```python
from build123d import *

# Parameters (mm, degrees)
F1_DEPTH  = 2
F3_DEPTH  = 3
F4_W      = 114.8
F4_H      = 24.2
F5_DEPTH  = 2
F7_DEPTH  = 2.2
F8_W      = 114.8
F8_H      = 2
F9_DEPTH  = 1
F10_W     = 114.8
F10_H     = 2
F11_DEPTH = 1
F12_DEPTH = 2


with BuildPart() as f1:
    # F0 (on Top) → F1 (new body)
    with BuildSketch(Plane.XY):
        Polygon((0, 40.2), (0, 0), (118.8, 0), (118.8, 40.2), (120.9, 40.2), (120.9, 155.2), (-2.1, 155.2), (-2.1, 40.2), align=None)
    extrude(amount=F1_DEPTH)

    # F2 (on face) → F3 (join)
    with BuildSketch(Plane.XY.offset(2)):
        Polygon((-2.1, 40.2), (0, 40.2), (0, 0), (118.8, 0), (118.8, 40.2), (120.9, 40.2), (120.9, 155.2), (-2.1, 155.2), align=None)
        Polygon((2, 42.2), (-0.1, 42.2), (-0.1, 153.2), (118.9, 153.2), (118.9, 42.2), (116.8, 42.2), (116.8, 2), (2, 2), align=None, mode=Mode.SUBTRACT)
    extrude(amount=F3_DEPTH)

    # F4 (on face) → F5 (join)
    with BuildSketch(Plane.XY.offset(2)):
        with Locations((59.4, 30.1)):
            Rectangle(F4_W, F4_H)
        Polygon((-0.1, 42.2), (2, 42.2), (59.4, 95.741176), (116.8, 42.2), (118.9, 42.2), (59.4, 97.7), align=None)
        Polygon((59.4, 97.7), (118.9, 42.2), (118.9, 44.158265), (61.499401, 97.7), (118.9, 151.241735), (118.9, 153.2), align=None)
        Polygon((-0.1, 153.2), (59.4, 97.7), (118.9, 153.2), (116.800599, 153.2), (59.4, 99.658265), (1.999401, 153.2), align=None)
        Polygon((-0.1, 44.158265), (-0.1, 42.2), (59.4, 97.7), (-0.1, 153.2), (-0.1, 151.241735), (57.300599, 97.7), align=None)
    extrude(amount=F5_DEPTH)

    # F6 (on face) → F7 (cut)
    with BuildSketch(Plane(origin=(0, 0, 0), x_dir=(1, 0, 0), z_dir=(0, 0, -1))):
        Polygon((0, -40.3), (118.8, -40.3), (118.8, -40.2), (118.8, -20.1), (0, -20.1), (0, -40.2), align=None)
    extrude(amount=-F7_DEPTH, mode=Mode.SUBTRACT)

    # F8 (on face) → F9 (cut)
    with BuildSketch(Plane.XY.offset(5)):
        with Locations((59.4, 1)):
            Rectangle(F8_W, F8_H)
    extrude(amount=-F9_DEPTH, mode=Mode.SUBTRACT)

    # F10 (on face) → F11 (cut)
    with BuildSketch(Plane.XY.offset(5)):
        with Locations((59.4, 154.2)):
            Rectangle(F10_W, F10_H)
    extrude(amount=-F11_DEPTH, mode=Mode.SUBTRACT)

    # F7_face (on face) → F12 (join)
    with BuildSketch(Plane(origin=(59.4, 97.748291, 0), x_dir=(1, 0, 0), z_dir=(0, 0, -1))):
        Polygon((-59.4, 57.548291), (-61.5, 57.548291), (-61.5, -57.451709), (61.5, -57.451709), (61.5, 57.548291), (59.4, 57.548291), (59.4, 57.448291), (-59.4, 57.448291), align=None)
    extrude(amount=F12_DEPTH)


solid = f1.part
```
Source: CAD feature listing. Evaluate the final solid. Frame: model axes, mm. A direction names the side the tool comes from. Round coordinates to 2 decimals unless told otherwise and drop trailing zeros. Loops run counter-clockwise (first coordinate to the right, second up) from the corner with the lowest first, then second, coordinate; pieces in that order, holes last. Notation, with made-up numbers: M 52.25,11.5 L 107.25,11.5 A33 ccw 107.25,41.5 Z; hole C -7.75,21 d9. An arc over 180 degrees is marked long. Use a Markdown table: item, result. Add a question column.
1. Reachability of faces 1 (the flat face through (88.5, 126.8, 3)), 2 (the flat face through (59, 30, 4)) from +Z, -Z, +X, -X, +Y, -Y: full face, straight path, thin tool, end or side. Return the list, or none.
2. Section query A-A on x = 94. Return the cut outline in (y, z), then the cut area to 3 significant figures.
3. Contact query for flat-ended pins moving along their axis: P1, Ø2.5, axis at y = 22, z = 3.5, coming from the -X side; P2, Ø0.6, axis at x = -1, z = 2, coming from the -Y side; P3, Ø10, axis at x = 73.5, y = 20, coming from the -Z side. Output: stop coordinate, or through.
4. Line query: line 1 (X direction, y = 125, z = 2.75); line 2 (Y direction, x = 91, z = 3); line 3 (X direction, y = 19, z = 4.75). Output: solid intervals per line, ascending.
5. Section query C-C on y = 47.5. Return the cut outline in (x, z).
6. Section query B-B on y = 137.5. Return the cut outline in (x, z), then the cut area to 3 significant figures.
7. Mould query, pull axis Y, two halves, no side actions, for faces 3 (the flat face through (59, 155.2, 1)), 4 (the flat face through (59, 10, 2)), 5 (the flat face through (-2.1, 97, 2)). Classes: pulls with the +Y half, pulls with the -Y half, needs draft (parallel to the pull), parting line crosses it, or undercut.
Reported:
| question | item | result |
|---|---|---|
| 1 | face 1 | +Z |
| 1 | face 2 | +Z, +Y, -Y |
| 2 | outline | M 0,0 L 20.1,0 L 20.1,2.2 L 40.3,2.2 L 40.3,-2 L 155.2,-2 L 155.2,4 L 153.2,4 L 153.2,2 L 131.93,2 L 131.93,4 L 128.02,4 L 128.02,2 L 67.38,2 L 67.38,4 L 63.47,4 L 63.47,2 L 42.2,2 L 42.2,4 L 18,4 L 18,2 L 2,2 L 2,4 L 0,4 Z |
| 2 | area | 568 mm² |
| 3 | P1 | stops at x = 0 |
| 3 | P2 | stops at y = 40.2 |
| 3 | P3 | stops at z = 0 |
| 4 | line 1 | x = -2.1 to -0.1, 28.03 to 32.23, 86.57 to 90.77, 118.9 to 120.9 |
| 4 | line 2 | y = 0 to 2, 18 to 42.2, 66.27 to 70.18, 125.22 to 129.13, 153.2 to 155.2 |
| 4 | line 3 | x = 0 to 2, 116.8 to 118.8 |
| 5 | outline | M -2.1,-2 L 120.9,-2 L 120.9,5 L 118.9,5 L 118.9,2 L 115.32,2 L 115.32,4 L 111.12,4 L 111.12,2 L 7.68,2 L 7.68,4 L 3.48,4 L 3.48,2 L -0.1,2 L -0.1,5 L -2.1,5 Z |
| 6 | outline | M -2.1,-2 L 120.9,-2 L 120.9,5 L 118.9,5 L 118.9,2 L 104.17,2 L 104.17,4 L 99.97,4 L 99.97,2 L 18.83,2 L 18.83,4 L 14.63,4 L 14.63,2 L -0.1,2 L -0.1,5 L -2.1,5 Z |
| 6 | area | 521 mm² |
| 7 | face 3 | pulls with the +Y half |
| 7 | face 4 | undercut |
| 7 | face 5 | needs draft |
